Verification items for the finished model (mm, model axes). A direction names the side the tool comes from. Round coordinates to 2 decimals unless told otherwise and drop trailing zeros. Write each loop counter-clockwise with the first axis right and the second up, starting at its lowest first coordinate (ties: lowest second). Pieces come first, ordered by that corner, then holes. Notation, with made-up numbers: M -28.75,70 L 25.25,70 A15 ccw 25.25,75 Z; hole C 16,35 d1. An arc over 180 degrees is marked long. One line per question, with ' | ' between items. Start each with the question number.
Q1. Thickness scan on line 1 along Y through (x, z) = (0.5, 1.25) (3 decimals); line 2 along Y through (x, z) = (-6.5, 2.25) (3 decimals); line 3 along X through (y, z) = (-11.5, -2). Record the ranges inside material, lowest first. Write a range as from..to.
Q2. Gauge pin test, flat end, axial feed: pin 1 (1.5 mm diameter, centred on y = 8.5, z = -1.5, fed in from -X). Record the tip position at first contact, or that the pin passes through.
Q3. Cross-section at B-B (x = 0). Record the boundary of the cut face in (y, z) (3 decimals), then the cut area to 3 significant figures.
Q4. Tool access check on faces 1 (the face through (0, -15, -3.969)), 2 (the face through (-12.3, -7.14, 0.06)). Record the directions out of +Z, -Z, +X, -X, +Y, -Y that give a thin tool (end or side, any length) a straight path to the whole face; none if there is none.
Q5. Cross-section at C-C (y = -19). Record the boundary of the cut face in (x, z).
Q6. Cross-section at A-A (y = 0). Record the boundary of the cut face in (x, z) (3 decimals), then the cut area to 3 significant figures.
Q7. Release check for a two-part mould opening along X. For faces 3 (the face through (0, -22.225, 0)), 4 (the face through (8.83, -15.14, 0.06)), 5 (the face through (0.581, 22.217, 0.056)) record: released by +X, released by -X, zero draft, split by the parting line, or undercut.
from build123d import *

# Parameters (mm, degrees)
BOSS_EXTRUDE1_DEPTH = 3.96875
FILLET2_R           = 2.032
FILLET3_R           = 9.525


with BuildPart() as part:
    # Sketch1 → Boss-Extrude1 (new, symmetric)
    with BuildSketch(Plane.XY):
        with BuildLine():
            Line((-21.258657525, -6.482291667), (-16.458315503, -22.225))
            Line((-16.458315503, -22.225), (16.458315503, -22.225))
            Line((16.458315503, -22.225), (21.258657525, -6.482291667))
            ThreePointArc((21.258657525, -6.482291667), (0, 22.225), (-21.258657525, -6.482291667))
        make_face()
        with BuildLine():
            ThreePointArc((13.55725, 4.303852743), (17.526, 0), (13.55725, -4.303852743))
            ThreePointArc((13.55725, -4.303852743), (12.318345343, -7.112), (10.50587081, -9.588996534))
            ThreePointArc((10.50587081, -9.588996534), (8.763, -15.177961227), (3.05137919, -13.892849277))
            ThreePointArc((3.05137919, -13.892849277), (0, -14.224), (-3.05137919, -13.892849277))
            ThreePointArc((-3.05137919, -13.892849277), (-8.763, -15.177961227), (-10.50587081, -9.588996534))
            ThreePointArc((-10.50587081, -9.588996534), (-12.318345343, -7.112), (-13.55725, -4.303852743))
            ThreePointArc((-13.55725, -4.303852743), (-17.526, 0), (-13.55725, 4.303852743))
            ThreePointArc((-13.55725, 4.303852743), (-12.318345343, 7.112), (-10.50587081, 9.588996534))
            ThreePointArc((-10.50587081, 9.588996534), (-8.763, 15.177961227), (-3.05137919, 13.892849277))
            ThreePointArc((-3.05137919, 13.892849277), (0, 14.224), (3.05137919, 13.892849277))
            ThreePointArc((3.05137919, 13.892849277), (8.763, 15.177961227), (10.50587081, 9.588996534))
            ThreePointArc((10.50587081, 9.588996534), (12.318345343, 7.112), (13.55725, 4.303852743))
        make_face(mode=Mode.SUBTRACT)
    extrude(amount=BOSS_EXTRUDE1_DEPTH, both=True)

    # Fillet2
    fillet2_edges = [part.edges().sort_by_distance(p)[0] for p in [
        (-13.55725, -4.303852743, 0),
        (-10.50587081, -9.588996534, 0),
        (-3.05137919, -13.892849277, 0),
        (3.05137919, -13.892849277, 0),
        (10.50587081, -9.588996534, 0),
        (13.55725, -4.303852743, 0),
        (13.55725, 4.303852743, 0),
        (10.50587081, 9.588996534, 0),
        (3.05137919, 13.892849277, 0),
        (-3.05137919, 13.892849277, 0),
        (-10.50587081, 9.588996534, 0),
        (-13.55725, 4.303852743, 0),
    ]]
    fillet(fillet2_edges, radius=FILLET2_R)

    # Fillet3
    fillet3_edges = [part.edges().sort_by_distance(p)[0] for p in [
        (16.458315503, -22.225, 0),
        (-16.458315503, -22.225, 0),
    ]]
    fillet(fillet3_edges, radius=FILLET3_R)


solid = part.part
Determined:
1) line 1: y = -22.225..-14.215, 14.215..22.219 | line 2: y = -22.225..-15.755, 15.755..21.253 | line 3: x = -19.73..-10.92, 10.92..19.73
2) pin 1: stops at x = -20.83
3) outline: M -22.225,-3.969 L -14.224,-3.969 L -14.224,3.969 L -22.225,3.969 Z; M 14.224,-3.969 L 22.225,-3.969 L 22.225,3.969 L 14.224,3.969 Z | area: 127 mm²
4) face 1: -Z, +X, -X, +Y, -Y | face 2: +Z, -Z
5) outline: M -16.55,-3.97 L 16.55,-3.97 L 16.55,3.97 L -16.55,3.97 Z
6) outline: M -22.225,-3.969 L -17.526,-3.969 L -17.526,3.969 L -22.225,3.969 Z; M 17.526,-3.969 L 22.225,-3.969 L 22.225,3.969 L 17.526,3.969 Z | area: 74.6 mm²
7) face 3: zero draft | face 4: undercut | face 5: split by the parting line
